```python
from build123d import *

# Parameters (mm, degrees)
CUT_EXTRUDE_1_DEPTH = 6.4


with BuildPart() as part:
    # Эскиз1 → Повернуть1 (revolve)
    with BuildSketch(Plane.XY, mode=Mode.PRIVATE) as revolve_1_sk:
        Polygon((5, 23), (5, 0), (22, 0), (22, 11), (11.27928518, 11), (11.27928518, 23), align=None)
    revolve(revolve_1_sk.sketch.rotate(Axis((0, 0, 0), (0, 1, 0)), 90), axis=Axis((0, 0, 0), (0, 1, 0)))

    # Эскиз2 → Вырез-Вытянуть1 (cut)
    with BuildSketch(Plane.XY):
        with BuildLine():
            Line((-1.5, 5), (-1.5, 20))
            ThreePointArc((-1.5, 20), (0, 21.5), (1.5, 20))
            Line((1.5, 20), (1.5, 5))
            ThreePointArc((1.5, 5), (0, 3.5), (-1.5, 5))
        make_face()
    extrude(amount=-CUT_EXTRUDE_1_DEPTH, mode=Mode.SUBTRACT)


solid = part.part
```
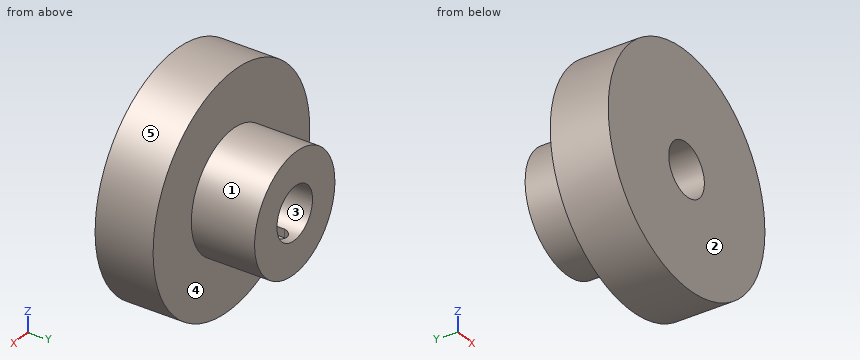
Model file for the job. Use its own axes, mm. Face numbers are marked on the shaded views. A direction names the side the tool comes from. Coordinates: 2 decimals unless noted, no trailing zeros. Loops run counter-clockwise (first coordinate to the right, second up) from the corner with the lowest first, then second, coordinate; pieces in that order, holes last. Notation, with made-up numbers: (-20, 59) - (24, 59) arc R23 ccw to (24, 94) - close; hole circle Ø2 at (65.5, 53). An arc over 180 degrees is marked (long way). Write item = value, one per line. Start each with the question number.
Item 1: Saw through at D-D, the plane x = 8.5. List the corners of the cut face in (y, z), then the cut area to 3 significant figures.
Item 2: Saw through at A-A, the plane z = 0. List the corners of the cut face in (x, y), then the cut area to 3 significant figures.
Item 3: Pull direction Z, two halves, no side cores. Call the marked faces 1, 2 and 3: +Z half, -Z half, draft (parallel to the pull), parting line (faces both ways), or undercut.
Item 4: Drop flat-ended pins along their axis: pin 1 Ø1 at (y, z) = (12.5, 14.5) entering from +X; pin 2 Ø1.8 at (y, z) = (9, -5.5) entering from -X; pin 3 Ø3 at (y, z) = (6, -14) entering from -X; pin 4 Ø10 at (x, z) = (-11, -16) entering from +Y. Give the stop position or say it passes through.
Item 5: Saw through at B-B, the plane y = 16.5. List the corners of the cut face in (x, z).
Item 6: 3-axis set-ups, long thin cutter, end or side, ignore diameter. For the marked faces 4 and 5: which of +Z, -Z, +X, -X, +Y, -Y reach the whole face in a straight line?
Item 7: Saw through at C-C, the plane x = 0. List the corners of the cut face in (y, z).
Item 8: Wall check: probe 1 along X at (y, z) = (13, 0); probe 2 along X at (y, z) = (7.5, 0); probe 3 along Y at (x, z) = (6.5, -20). Give the ranges that are in metal, low to high. Write a range as [from, to].
Answers:
q1.outline = (0, -20.29) - (11, -20.29) - (11, -7.41) - (23, -7.41) - (23, 7.41) - (11, 7.41) - (11, 20.29) - (0, 20.29) - close
q1.area = 624 mm2
q2.outline = (-22, 0) - (-5, 0) - (-5, 23) - (-11.28, 23) - (-11.28, 11) - (-22, 11) - close; (5, 0) - (22, 0) - (22, 11) - (11.28, 11) - (11.28, 23) - (5, 23) - close
q2.area = 525 mm2
q3.face_1 = parting line
q3.face_2 = draft
q3.face_3 = undercut
q4.pin_1 = through
q4.pin_2 = -21.51
q4.pin_3 = -18.1
q4.pin_4 = 11
q5.outline = circle Ø22.56 at (0, 0); hole (-1.5, -6.4) - (1.5, -6.4) - (1.5, -4.77) arc R5 ccw (long way) to (-1.5, -4.77) - close
q6.face_4 = +Y
q6.face_5 = +Y, -Y
q7.outline = (0, -22) - (11, -22) - (11, -11.28) - (23, -11.28) - (23, -5) - (21.5, -5) - (21.5, -6.4) - (3.5, -6.4) - (3.5, -5) - (0, -5) - close; (0, 5) - (23, 5) - (23, 11.28) - (11, 11.28) - (11, 22) - (0, 22) - close
q8.probe_1 = [-11.28, -5], [5, 11.28]
q8.probe_2 = [-22, -5], [5, 22]
q8.probe_3 = [0, 11]
